```python
from build123d import *

# Parameters (mm, degrees)
EXTRUDE_1_DEPTH     = 1.6
SKETCH_3_W          = 84
SKETCH_3_H          = 26.4
EXTRUDE_1_2_DEPTH   = 2.8
CUT_EXTRUDE_1_DEPTH = 1.2
SKETCH_8_R          = 2.35345012
EXTRUDE_2_DEPTH     = 4.4
CUT_EXTRUDE_2_DEPTH = 0.2
FILLET_2_R          = 0.4
SKETCH_10_W         = 2.4
SKETCH_10_H         = 27.704592787
SKETCH_10_H_2       = 28.279400909
CUT_EXTRUDE_3_DEPTH = 12
SKETCH_11_R         = 1.3
CUT_EXTRUDE_4_DEPTH = 12
CHAMFER_1_SIZE      = 0.8
SKETCH_12_R         = 1.5
CUT_EXTRUDE_5_DEPTH = 12
SKETCH_13_R         = 3
CUT_EXTRUDE_6_DEPTH = 12
CUT_EXTRUDE_7_DEPTH = 1.2
SKETCH_15_R         = 1.5
EXTRUDE_4_DEPTH     = 1.6


with BuildPart() as part:
    # Эскиз2 → Extrude 1 (new body)
    with BuildSketch(Plane.XY):
        with BuildLine():
            Line((45.6, -13.6), (45.6, -7.203828964))
            Line((45.6, -7.203828964), (45.6, 7.296171036))
            Line((45.6, 7.296171036), (45.6, 16.8))
            Line((45.6, 16.8), (42.6, 16.8))
            Line((42.6, 16.8), (39.6, 16.8))
            Line((39.6, 16.8), (-39.6, 16.8))
            Line((-39.6, 16.8), (-42.6, 16.8))
            Line((-42.6, 16.8), (-45.6, 16.8))
            Line((-45.6, 16.8), (-45.6, -13.6))
            ThreePointArc((-45.6, -13.6), (-44.6627417, -15.8627417), (-42.4, -16.8))
            Line((-42.4, -16.8), (42.4, -16.8))
            ThreePointArc((42.4, -16.8), (44.6627417, -15.8627417), (45.6, -13.6))
        make_face()
    extrude(amount=EXTRUDE_1_DEPTH)

    # Эскиз3 → Extrude 1 2 (add)
    with BuildSketch(Plane.XY.offset(1.6)):
        with BuildLine():
            Line((-42.2, -15), (42.2, -15))
            ThreePointArc((42.2, -15), (43.33137085, -14.53137085), (43.8, -13.4))
            Line((43.8, -13.4), (43.8, 13.4))
            ThreePointArc((43.8, 13.4), (43.33137085, 14.53137085), (42.2, 15))
            Line((42.2, 15), (-42.2, 15))
            ThreePointArc((-42.2, 15), (-43.33137085, 14.53137085), (-43.8, 13.4))
            Line((-43.8, 13.4), (-43.8, -13.4))
            ThreePointArc((-43.8, -13.4), (-43.33137085, -14.53137085), (-42.2, -15))
        make_face()
        Rectangle(SKETCH_3_W, SKETCH_3_H, mode=Mode.SUBTRACT)
    extrude(amount=-EXTRUDE_1_2_DEPTH)

    # Эскиз4 → Вырез-Вытянуть-Тонкостенный1 (cut)
    with BuildSketch(Plane(origin=(0, 0, -1.2), x_dir=(-1, 0, 0), z_dir=(0, 0, -1))):
        with BuildLine():
            Line((-43.8, 13.4), (-43.8, -13.4))
            ThreePointArc((-43.8, -13.4), (-43.33137085, -14.53137085), (-42.2, -15))
            Line((-42.2, -15), (42.2, -15))
            ThreePointArc((42.2, -15), (43.33137085, -14.53137085), (43.8, -13.4))
            Line((43.8, -13.4), (43.8, 13.4))
            ThreePointArc((43.8, 13.4), (43.33137085, 14.53137085), (42.2, 15))
            Line((42.2, 15), (-42.2, 15))
            ThreePointArc((-42.2, 15), (-43.33137085, 14.53137085), (-43.8, 13.4))
        make_face()
        with BuildLine():
            Line((-43.2, 13.4), (-43.2, -13.4))
            ThreePointArc((-43.2, -13.4), (-42.907106781, -14.107106781), (-42.2, -14.4))
            Line((-42.2, -14.4), (42.2, -14.4))
            ThreePointArc((42.2, -14.4), (42.907106781, -14.107106781), (43.2, -13.4))
            Line((43.2, -13.4), (43.2, 13.4))
            ThreePointArc((43.2, 13.4), (42.907106781, 14.107106781), (42.2, 14.4))
            Line((42.2, 14.4), (-42.2, 14.4))
            ThreePointArc((-42.2, 14.4), (-42.907106781, 14.107106781), (-43.2, 13.4))
        make_face(mode=Mode.SUBTRACT)
    extrude(amount=-CUT_EXTRUDE_1_DEPTH, mode=Mode.SUBTRACT)

    # Эскиз8 → Бобышка-Вытянуть2 (add)
    with BuildSketch(Plane(origin=(0, 0, 0), x_dir=(-1, 0, 0), z_dir=(0, 0, -1))):
        with Locations((-41.44654988, 12.046171036)):
            Circle(SKETCH_8_R)
        with Locations((-41.44654988, -11.953828964)):
            Circle(SKETCH_8_R)
        with Locations((41.1, 12.046171036)):
            Circle(SKETCH_8_R)
        with Locations((41.1, -11.953828964)):
            Circle(SKETCH_8_R)
    extrude(amount=EXTRUDE_2_DEPTH)

    # Эскиз9 → Вырез-Вытянуть2 (cut)
    with BuildSketch(Plane(origin=(0, 0, 0), x_dir=(-1, 0, 0), z_dir=(0, 0, -1))):
        with BuildLine():
            Line((-44.8, -6.403828964), (-44.8, 6.496171036))
            ThreePointArc((-44.8, 6.496171036), (-45.365685425, 6.730485611), (-45.6, 7.296171036))
            Line((-45.6, 7.296171036), (-45.6, -7.203828964))
            ThreePointArc((-45.6, -7.203828964), (-45.365685425, -6.638143539), (-44.8, -6.403828964))
        make_face()
    extrude(amount=-CUT_EXTRUDE_2_DEPTH, mode=Mode.SUBTRACT)

    # Скругление2
    fillet_2_edges = [part.edges().sort_by_distance(p)[0] for p in [
        (45.6, 0.046171036, 0.2),
    ]]
    fillet(fillet_2_edges, radius=FILLET_2_R)

    # Эскиз10 → Вырез-Вытянуть3 (cut)
    with BuildSketch(Plane(origin=(0, 0, 0), x_dir=(-1, 0, 0), z_dir=(0, 0, -1))):
        with Locations((-44.4, 0.252296393)):
            Rectangle(SKETCH_10_W, SKETCH_10_H)
        with Locations((44.4, 0.539700455)):
            Rectangle(SKETCH_10_W, SKETCH_10_H_2)
    extrude(amount=CUT_EXTRUDE_3_DEPTH, mode=Mode.SUBTRACT)

    # Эскиз11 → Вырез-Вытянуть4 (cut)
    with BuildSketch(Plane(origin=(0, 0, -4.4), x_dir=(-1, 0, 0), z_dir=(0, 0, -1))):
        with Locations((-41.44654988, 12.046171036)):
            Circle(SKETCH_11_R)
        with Locations((-41.44654988, -11.953828964)):
            Circle(SKETCH_11_R)
        with Locations((41.1, -11.953828964)):
            Circle(SKETCH_11_R)
        with Locations((41.1, 12.046171036)):
            Circle(SKETCH_11_R)
    extrude(amount=-CUT_EXTRUDE_4_DEPTH, mode=Mode.SUBTRACT)

    # Фаска1
    chamfer_1_edges = [part.edges().sort_by_distance(p)[0] for p in [
        (-39.8, 12.046171036, 1.6),
        (-39.8, -11.953828964, 1.6),
        (42.74654988, -11.953828964, 1.6),
        (42.74654988, 12.046171036, 1.6),
    ]]
    chamfer(chamfer_1_edges, length=CHAMFER_1_SIZE)

    # Эскиз12 → Вырез-Вытянуть5 (cut)
    with BuildSketch(Plane(origin=(0, 0, 0), x_dir=(-1, 0, 0), z_dir=(0, 0, -1))):
        with Locations((-35, -6.2)):
            Circle(SKETCH_12_R)
        with Locations((-25, -6.2)):
            Circle(SKETCH_12_R)
        with Locations((-15, -6.2)):
            Circle(SKETCH_12_R)
        with Locations((-5, -6.2)):
            Circle(SKETCH_12_R)
        with Locations((5, -6.2)):
            Circle(SKETCH_12_R)
        with Locations((15, -6.2)):
            Circle(SKETCH_12_R)
        with Locations((25, -6.2)):
            Circle(SKETCH_12_R)
        with Locations((35, -6.2)):
            Circle(SKETCH_12_R)
    extrude(amount=-CUT_EXTRUDE_5_DEPTH, mode=Mode.SUBTRACT)

    # Эскиз13 → Вырез-Вытянуть6 (cut)
    with BuildSketch(Plane(origin=(0, 0, 0), x_dir=(-1, 0, 0), z_dir=(0, 0, -1))):
        with Locations((-39.94654988, -5.953828964)):
            Circle(SKETCH_13_R)
        Polygon((-42.94654988, 9.046171036), (-36.94654988, 9.046171036), (-39.94654988, 3.850018614), align=None)
    extrude(amount=-CUT_EXTRUDE_6_DEPTH, mode=Mode.SUBTRACT)

    # Эскиз14 → Вырез-Вытянуть7 (cut)
    with BuildSketch(Plane(origin=(0, 0, -1.2), x_dir=(-1, 0, 0), z_dir=(0, 0, -1))):
        with BuildLine():
            Line((-42, -9.666380509), (-42, 9.758722582))
            ThreePointArc((-42, 9.758722582), (-42.654530459, 10.026391249), (-43.2, 10.476413047))
            Line((-43.2, 10.476413047), (-43.2, -10.384070975))
            ThreePointArc((-43.2, -10.384070975), (-42.654530459, -9.934049177), (-42, -9.666380509))
        make_face()
    extrude(amount=-CUT_EXTRUDE_7_DEPTH, mode=Mode.SUBTRACT)

    # Эскиз15 → Бобышка-Вытянуть4 (add)
    with BuildSketch(Plane(origin=(0, 0, 0), x_dir=(-1, 0, 0), z_dir=(0, 0, -1))):
        with Locations((35, -6.2)):
            Circle(SKETCH_15_R)
        with Locations((-35, -6.2)):
            Circle(SKETCH_15_R)
    extrude(amount=-EXTRUDE_4_DEPTH)


solid = part.part
```
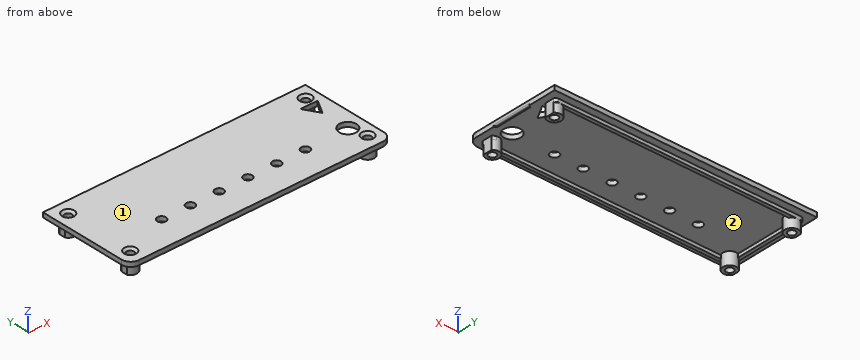
Input: part model. Units: mm. Frame: model coordinates. Face numbers are marked on the shaded views. Round coordinates to 2 decimals unless told otherwise and drop trailing zeros. Loops run counter-clockwise (first coordinate to the right, second up) from the corner with the lowest first, then second, coordinate; pieces in that order, holes last.
1) Section query A-A on x = -41.1. Count the separate pieces of the cut face and the enclosed holes in it, plus the area to 3 significant figures.
Ans:
separate pieces: 3
enclosed holes: 0
area: 62.8 mm2
2) Section query B-B on x = 25. Return the cut outline in (y, z).
Ans:
outline: (-16.8, 0) - (-14.4, 0) - (-14.4, -1.2) - (-13.2, -1.2) - (-13.2, 0) - (-7.7, 0) - (-7.7, 1.6) - (-16.8, 1.6) - close; (-4.7, 0) - (13.2, 0) - (13.2, -1.2) - (14.4, -1.2) - (14.4, 0) - (16.8, 0) - (16.8, 1.6) - (-4.7, 1.6) - close
3) Material intervals for line 1 (X direction, y = 12, z = -1.5); line 2 (Y direction, x = 22, z = -0.5); line 3 (Y direction, x = -39, z = -2.5), sorted ascending.
Ans:
line 1: x = -43.2 to -42.4, -39.8 to -38.75, 39.09 to 40.15, 42.75 to 43.2
line 2: y = -14.4 to -13.2, 13.2 to 14.4
line 3: y = -13.02 to -10.89, 10.98 to 13.11
4) Section query C-C on z = -2.25. Return the cut outline in (x, y), plus the area to 3 significant figures.
Ans:
outline: (-43.2, -13.02) arc R2.35 ccw (long way) to (-43.2, -10.89) - close; (-43.2, 10.98) arc R2.35 ccw (long way) to (-43.2, 13.11) - close; (43.2, -13.52) - (43.2, -10.38) arc R2.35 ccw (long way) to start; (43.2, 10.48) - (43.2, 13.62) arc R2.35 ccw (long way) to start; hole circle Ø2.6 at (-41.1, -11.95); hole circle Ø2.6 at (-41.1, 12.05); hole circle Ø2.6 at (41.45, -11.95); hole circle Ø2.6 at (41.45, 12.05)
area: 45.1 mm2
5) Pull-direction query (Y, two-part tool) for the marked faces 1 and 2; classes: released by +Y, released by -Y, zero draft, split by the parting line, or undercut.
Ans:
face 1: zero draft
face 2: undercut
6) Pin query (flat end, axial travel): pin 1 (5 mm diameter, centred on x = -15, y = -6.2, fed in from -Z); pin 2 (5.5 mm diameter, centred on x = 39.95, y = -5.95, fed in from -Z); pin 3 (0.6 mm diameter, centred on x = -4.5, z = -0.5, fed in from -Y); pin 4 (2 mm diameter, centred on y = -6.5, z = 0, fed in from +X). Return the tip coordinate at first contact, or that it passes through.
Ans:
pin 1: stops at z = 0
pin 2: passes through
pin 3: stops at y = -14.4
pin 4: stops at x = 45.6
